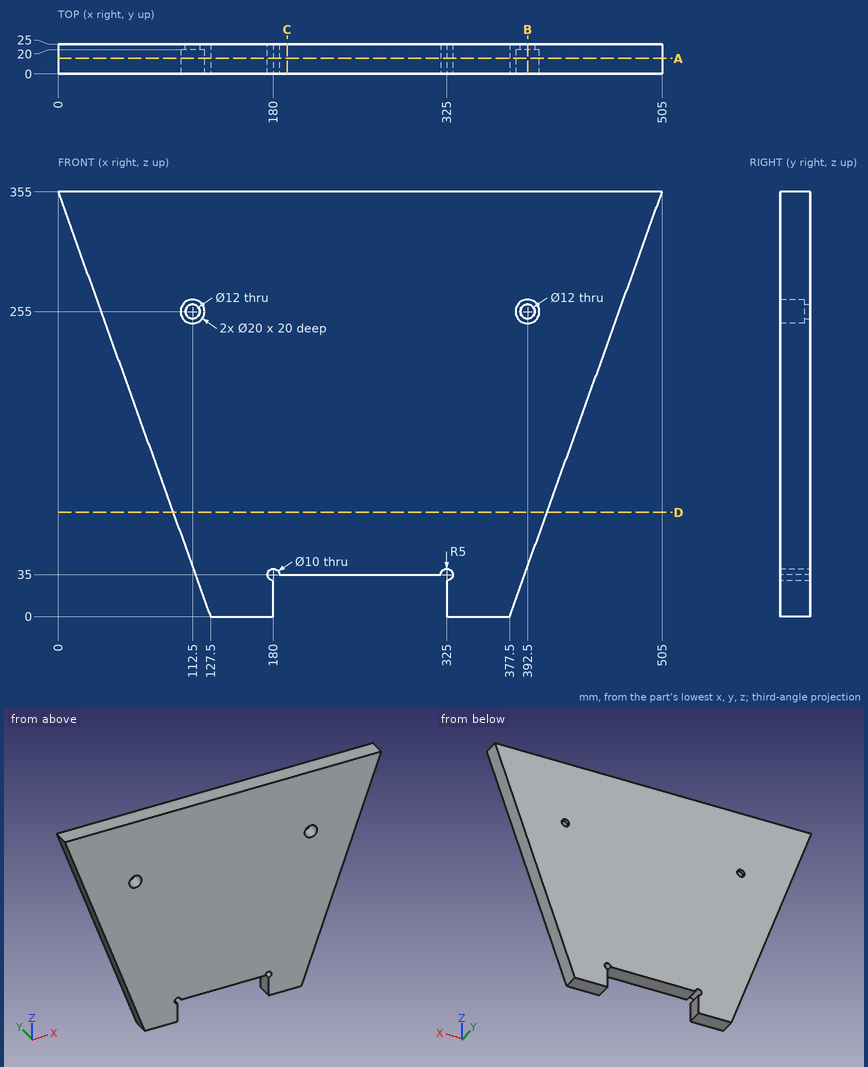
Here's the drawing with two shaded views (mm, measured from the low corner). I have some questions. Coordinates: 2 decimals unless noted, no trailing zeros. Loops run counter-clockwise (first coordinate to the right, second up) from the corner with the lowest first, then second, coordinate; pieces in that order, holes last. Notation, with made-up numbers: M -9,19.5 L 26,19.5 A26 cw 26,33.5 Z; hole C 39,9.25 d11. An arc over 180 degrees is marked long. Answer as CSV lines item,"result". Start each with the question number.
1. For pin 1 Ø15.5 at (x, z) = (392.5, 255) entering from -Y; pin 2 Ø6 at (x, z) = (180, 35) entering from +Y; pin 3 Ø3 at (y, z) = (5.5, 115.5) entering from +X; pin 4 Ø12 at (y, z) = (11.5, 184.5) entering from -X, each with a flat end and sliding along its axis, tell me the tip position at first contact or that it passes through.
2. Suppose I cut it at A-A, the plane y = 13. List the corners of the cut face in (x, z) for me, plus the area to 3 significant figures.
3. Suppose I cut it at B-B, the plane x = 392.5. List the corners of the cut face in (y, z) for me.
4. Suppose I cut it at D-D, the plane z = 87. List the corners of the cut face in (x, y) for me, plus the area to 3 significant figures.
5. If I drill on probe 1 along X at (y, z) = (21.05, 255); probe 2 along X at (y, z) = (9.25, 251); probe 3 along Z at (x, y) = (221.5, 12.5), over which ranges is the centre line in solid material (lowest first)? Write a range as [from, to].
6. Suppose I cut it at C-C, the plane x = 191.5. List the corners of the cut face in (y, z) for me.
Output:
1,pin 1,"stops at y = 20"
1,pin 2,"passes through"
1,pin 3,"stops at x = 419.52"
1,pin 4,"stops at x = 59.08"
2,outline,"M 0,355 L 127.5,0 L 180,0 L 180,30 A5 cw long 185,35 L 320,35 A5 cw long 325,30 L 325,0 L 377.5,0 L 505,355 Z; hole C 112.5,255 d20; hole C 392.5,255 d20"
2,area,"128,000 mm^2"
3,outline,"M 0,41.76 L 25,41.76 L 25,249 L 20,249 L 20,245 L 0,245 Z; M 0,265 L 20,265 L 20,261 L 25,261 L 25,355 L 0,355 Z"
4,outline,"M 96.25,0 L 408.75,0 L 408.75,25 L 96.25,25 Z"
4,area,"7,810 mm^2"
5,probe 1,"x = [35.92, 106.5], [118.5, 386.5], [398.5, 469.08]"
5,probe 2,"x = [37.35, 103.33], [121.67, 383.33], [401.67, 467.65]"
5,probe 3,"z = [35, 355]"
6,outline,"M 0,35 L 25,35 L 25,355 L 0,355 Z"
